from build123d import *

# Parameters (mm, degrees)
BOSS_EXTRUDE1_DEPTH = 12
FILLET1_R           = 2
SKETCH3_W           = 8
SKETCH3_H           = 14
CUT_EXTRUDE1_DEPTH  = 33.407560846
FILLET5_R           = 1
SKETCH4_R           = 1.65
CUT_EXTRUDE2_DEPTH  = 30.295904151
SKETCH6_R           = 0.5
CUT_EXTRUDE3_DEPTH  = 54


with BuildPart() as part:
    # Sketch2 → Boss-Extrude1 (new body)
    with BuildSketch(Plane.XY):
        with BuildLine():
            Line((-8, -17.5), (-8, 17.5))
            ThreePointArc((-8, 17.5), (0, 25.5), (8, 17.5))
            Line((8, 17.5), (8, -17.5))
            ThreePointArc((8, -17.5), (0, -25.5), (-8, -17.5))
        make_face()
    extrude(amount=BOSS_EXTRUDE1_DEPTH)

    # Fillet1
    fillet1_edges = [part.edges().sort_by_distance(p)[0] for p in [
        (0, 25.5, 12),
        (-8, 0, 12),
        (0, -25.5, 12),
        (-8, 0, 0),
        (0, 25.5, 0),
        (8, 0, 0),
        (0, -25.5, 0),
        (8, 0, 12),
    ]]
    fillet(fillet1_edges, radius=FILLET1_R)

    # Sketch3 → Cut-Extrude1 (cut, through all)
    with BuildSketch(Plane(origin=(8, 0, 0), x_dir=(0, 0, -1), z_dir=(1, 0, 0))):
        with Locations((-6, 18.5)):
            Rectangle(SKETCH3_W, SKETCH3_H)
    extrude(amount=-CUT_EXTRUDE1_DEPTH, mode=Mode.SUBTRACT)

    # Fillet5
    fillet5_edges = [part.edges().sort_by_distance(p)[0] for p in [
        (0, 11.5, 10),
        (0, 11.5, 2),
    ]]
    fillet(fillet5_edges, radius=FILLET5_R)

    # Sketch4 → Cut-Extrude2 (cut, through all)
    with BuildSketch(Plane.XY.offset(12)):
        with Locations((0, 17)):
            Circle(SKETCH4_R)
        with Locations((0, -20)):
            Circle(SKETCH4_R)
    extrude(amount=-CUT_EXTRUDE2_DEPTH, mode=Mode.SUBTRACT)

    # Sketch6 → Cut-Extrude3 (cut, through all)
    with BuildSketch(Plane(origin=(0, -25.5, 0), x_dir=(-1, 0, 0), z_dir=(0, -1, 0))):
        with Locations(Location((-5.5, -6, 0), (0, 0, 90))):
            Circle(SKETCH6_R)
        with Locations(Location((5.5, -6, 0), (0, 0, 90))):
            Circle(SKETCH6_R)
    extrude(amount=-CUT_EXTRUDE3_DEPTH, mode=Mode.SUBTRACT)


solid = part.part
CAD build for the part. Positions are in the model's coordinates, mm. A direction names the side the tool comes from. Round coordinates to 2 decimals unless told otherwise and drop trailing zeros. Write each loop counter-clockwise with the first axis right and the second up, starting at its lowest first coordinate (ties: lowest second). Pieces come first, ordered by that corner, then holes. Notation, with made-up numbers: M 60.25,-20.75 L 91.25,-20.75 A35 cw 91.25,17.25 Z; hole C -33,-7.5 d10. An arc over 180 degrees is marked long. Use a Markdown table: item, result. Add a question column.
1. Slice it at A-A on y = 17. Give the cut face in (x, z), then the cut area to 3 significant figures.
2. 3-axis set-ups, long thin cutter, end or side, ignore diameter. For faces 5 (the face through (0, 0, 12)), 6 (the face through (-0.112, 11.801, 9.715)): which of +Z, -Z, +X, -X, +Y, -Y reach the whole face in a straight line?
3. Slice it at B-B on x = 0. Give the cut face in (y, z).
4. Slice it at C-C on y = -16. Give the cut face in (x, z).
5. Flat gauge pins, fed straight in: P1, Ø3, axis at x = 1, z = 6, coming from the +Y side; P2, Ø3, axis at y = 15, z = 5, coming from the +X side. Where does each tip first touch, or does it go through?
6. Pull direction Y, two halves, no side cores. Call faces 1 (the face through (-0.112, 11.801, 2.285)), 2 (the face through (0.89, 18.39, 1.01)), 3 (the face through (-0.215, -18.364, 6.084)), 4 (the face through (-5, -6, 6)): released by +Y, released by -Y, zero draft, split by the parting line, or undercut.
7. Drill centre lines: probe 1 along X at (y, z) = (1.5, 6); probe 2 along Z at (x, y) = (-2, 19); probe 3 along Y at (x, z) = (0, 11.1). Where is each one in solid material? Low to high.
8. Slice it at D-D on z = 5. Give the cut face in (x, y).
Reply:
| question | item | result |
|---|---|---|
| 1 | outline | M -8,2 A2 ccw -6,0 L -1.65,0 L -1.65,2 Z; M -8,10 L -1.65,10 L -1.65,12 L -6,12 A2 ccw Z; M 1.65,0 L 6,0 A2 ccw 8,2 L 1.65,2 Z; M 1.65,10 L 8,10 A2 ccw 6,12 L 1.65,12 Z |
| 1 | area | 47.4 mm^2 |
| 2 | face 5 | +Z, +X, -X, +Y, -Y |
| 2 | face 6 | +X, -X, +Y |
| 3 | outline | M -25.5,2 A2 ccw -23.5,0 L -21.65,0 L -21.65,12 L -23.5,12 A2 ccw -25.5,10 Z; M -18.35,0 L 15.35,0 L 15.35,2 L 12.5,2 A1 cw 11.5,3 L 11.5,9 A1 cw 12.5,10 L 15.35,10 L 15.35,12 L -18.35,12 Z; M 18.65,0 L 23.5,0 A2 ccw 25.5,2 L 18.65,2 Z; M 18.65,10 L 25.5,10 A2 ccw 23.5,12 L 18.65,12 Z |
| 4 | outline | M -8,2 A2 ccw -6,0 L 6,0 A2 ccw 8,2 L 8,10 A2 ccw 6,12 L -6,12 A2 ccw -8,10 Z; hole C -5.5,6 d1; hole C 5.5,6 d1 |
| 5 | P1 | stops at y = 11.5 |
| 5 | P2 | passes through |
| 6 | face 1 | released by +Y |
| 6 | face 2 | undercut |
| 6 | face 3 | undercut |
| 6 | face 4 | zero draft |
| 7 | probe 1 | x = -8 to -6, -5 to 5, 6 to 8 |
| 7 | probe 2 | z = 0 to 2, 10 to 12 |
| 7 | probe 3 | y = -25.17 to -21.65, -18.35 to 15.35, 18.65 to 25.17 |
| 8 | outline | M -8,-17.5 A8 ccw 8,-17.5 L 8,11.5 L -8,11.5 Z; hole C 0,-20 d3.3 |
